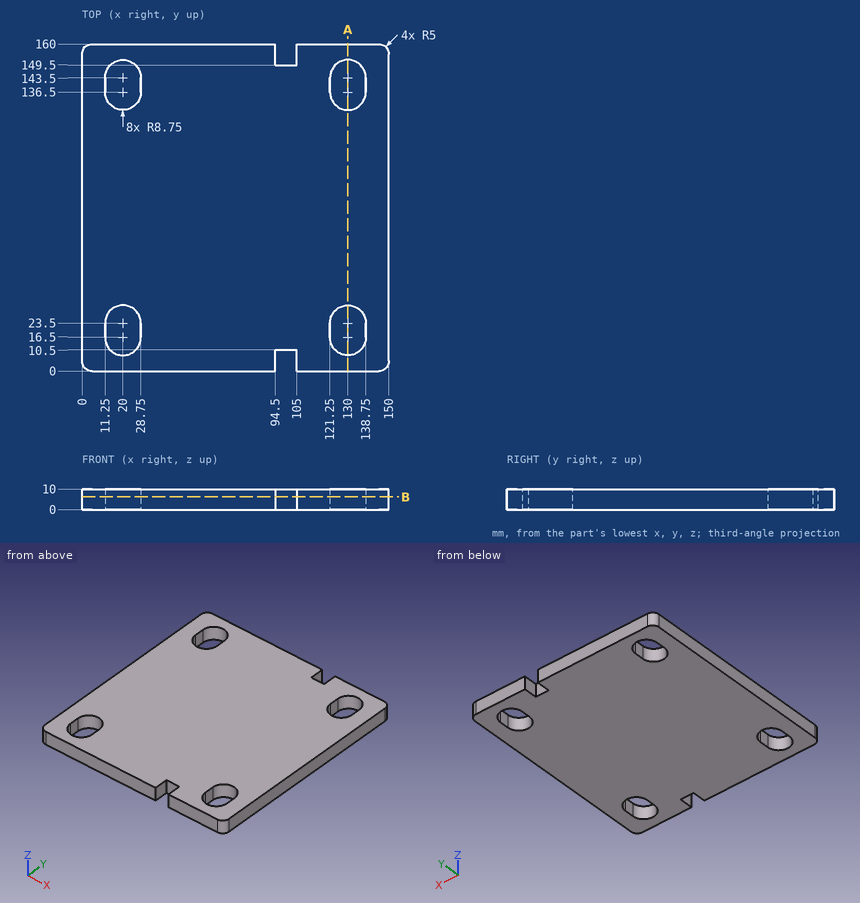
Can you work these out from the drawing? Everything is in mm from the part's minimum corner. Coordinates: 2 decimals unless noted, no trailing zeros. Loops run counter-clockwise (first coordinate to the right, second up) from the corner with the lowest first, then second, coordinate; pieces in that order, holes last. Notation, with made-up numbers: M 54,32 L 108,32 A29 ccw 108,52 Z; hole C 67,87 d11. An arc over 180 degrees is marked long. One line per item, written item: value.
1. Imagine slicing it at B-B (z = 6.25). State how many separate pieces and enclosed holes the cut face has, and give its area (3 significant figures).
Geometry says:
separate pieces: 1
enclosed holes: 4
area: 22,300 mm2
2. Imagine slicing it at A-A (x = 130). List the corners of the cut face in (y, z) for me, and give its area (3 significant figures).
Geometry says:
outline: M 0,0 L 7.75,0 L 7.75,10 L 0,10 Z; M 32.25,0 L 127.75,0 L 127.75,10 L 32.25,10 Z; M 152.25,0 L 160,0 L 160,10 L 152.25,10 Z
area: 1,110 mm2
3. Please list where these lines run through material, in increasing order: probe 1 along X at (y, z) = (144, 9); probe 2 along X at (y, z) = (137, 7.25); probe 3 along Y at (x, z) = (14, 4.25).
Geometry says:
probe 1: x = 0 to 11.26, 28.74 to 121.26, 138.74 to 150
probe 2: x = 0 to 11.25, 28.75 to 121.25, 138.75 to 150
probe 3: y = 0 to 10.13, 29.87 to 130.13, 149.87 to 160
4. Will this pin go through, and if not, where does the flat tip stop? pin 1 Ø5 at (x, z) = (101.5, 3) entering from +Y.
Geometry says:
pin 1: stops at y = 149.5
